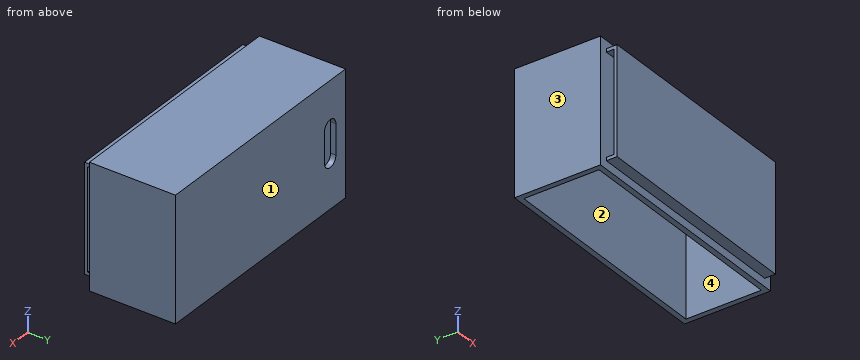
```python
from build123d import *

# Parameters (mm, degrees)
SKETCH3_W           = 55.88
SKETCH3_H           = 29.21
BOSS_EXTRUDE4_DEPTH = 20.32
SKETCH5_W           = 53.34
SKETCH5_H           = 17.78
CUT_EXTRUDE1_DEPTH  = 27.94
CUT_EXTRUDE2_REACH  = 22.32
SKETCH7_W           = 52.07
SKETCH7_H           = 25.4
BOSS_EXTRUDE5_DEPTH = 2.54
CUT_EXTRUDE3_REACH  = 55.975
SKETCH8_W           = 23.876
SKETCH8_H           = 1.778


with BuildPart() as part:
    # Sketch3 → Boss-Extrude4 (new body)
    with BuildSketch(Plane(origin=(0, 0, 0), x_dir=(1, 0, 0), z_dir=(0, 1, 0))):
        with Locations((27.94, 14.605)):
            Rectangle(SKETCH3_W, SKETCH3_H)
    extrude(amount=BOSS_EXTRUDE4_DEPTH)

    # Sketch5 → Cut-Extrude1 (cut)
    with BuildSketch(Plane(origin=(0, 0, -29.21), x_dir=(-1, 0, 0), z_dir=(0, 0, -1))):
        with Locations((-27.94, 10.16)):
            Rectangle(SKETCH5_W, SKETCH5_H)
    extrude(amount=-CUT_EXTRUDE1_DEPTH, mode=Mode.SUBTRACT)

    # Sketch6 → Cut-Extrude2 (cut, up to next)
    with BuildSketch(Plane(origin=(0, 20.32, 0), x_dir=(1, 0, 0), z_dir=(0, 1, 0)), mode=Mode.PRIVATE) as cut_extrude2_sk1:
        with BuildLine():
            Line((6.891061211, 17.925123576), (6.891061211, 10.769129072))
            ThreePointArc((6.891061211, 10.769129072), (5.021477061, 8.899544922), (3.151892912, 10.769129072))
            Line((3.151892912, 10.769129072), (3.151892912, 17.925123576))
            ThreePointArc((3.151892912, 17.925123576), (5.021477061, 19.794707726), (6.891061211, 17.925123576))
        make_face()
    cut_extrude2_tool1 = extrude(cut_extrude2_sk1.sketch, amount=-CUT_EXTRUDE2_REACH, mode=Mode.PRIVATE) & part.part
    add(cut_extrude2_tool1.solids().sort_by_distance((5.021477, 20.32, -14.347126))[0], mode=Mode.SUBTRACT)

    # Sketch7 → Boss-Extrude5 (add)
    with BuildSketch(Plane.XZ):
        with Locations((27.94, -14.605)):
            Rectangle(SKETCH7_W, SKETCH7_H)
    extrude(amount=BOSS_EXTRUDE5_DEPTH)

    # Sketch8 → Cut-Extrude3 (cut, up to next)
    with BuildSketch(Plane.ZY.offset(-1.905), mode=Mode.PRIVATE) as cut_extrude3_sk1:
        with Locations((-14.605, -0.889)):
            Rectangle(SKETCH8_W, SKETCH8_H)
    cut_extrude3_tool1 = extrude(cut_extrude3_sk1.sketch, amount=-CUT_EXTRUDE3_REACH, mode=Mode.PRIVATE) & part.part
    add(cut_extrude3_tool1.solids().sort_by_distance((1.905, -0.889, -14.605))[0], mode=Mode.SUBTRACT)


solid = part.part
```
The model under review builds one solid part; all positions refer to its coordinate system, in mm. Face numbers are marked on the shaded views. Round coordinates to 2 decimals unless told otherwise and drop trailing zeros. Order: outer loops, then holes, each group sorted by start corner. A loop starts at its lowest first (then second) coordinate and runs counter-clockwise, first axis right, second up. Notation, with made-up numbers: (34.5, 13.5) -> (84.5, 13.5) arc R20 ccw to (84.5, 23.5) -> close; hole circle Ø6 at (-34, 35.5). An arc over 180 degrees is marked (long way). Use a Markdown table: item, result.
Q1. Mouldability with a two-part tool opening along Y and no side actions: class the marked faces 1, 2, 3 and 4 as +Y half, -Y half, draft (parallel to the pull), parting line (faces both ways), or undercut.
Values:
| item | result |
|---|---|
| face 1 | +Y half |
| face 2 | undercut |
| face 3 | draft |
| face 4 | undercut |
Q2. We need section A-A on z = -5.25. Write out the cut boundary in (x, y) (3 decimals).
Values:
| item | result |
|---|---|
| outline | (0, 0) -> (55.88, 0) -> (55.88, 20.32) -> (0, 20.32) -> close; (1.905, -2.54) -> (53.975, -2.54) -> (53.975, -1.778) -> (1.905, -1.778) -> close; hole (1.27, 1.27) -> (54.61, 1.27) -> (54.61, 19.05) -> (1.27, 19.05) -> close |
Q3. For line 1 (Y direction, x = 38.5, z = -19.75); line 2 (X direction, y = 13.75, z = -18); line 3 (Y direction, x = 22.5, z = -1), list the stretches that pass through material, from the lowest coordinate up.
Values:
| item | result |
|---|---|
| line 1 | y = -2.54 to -1.78, 0 to 1.27, 19.05 to 20.32 |
| line 2 | x = 0 to 1.27, 54.61 to 55.88 |
| line 3 | y = 0 to 20.32 |
Q4. We need section C-C on z = -12.5. Write out the cut boundary in (x, y) (3 decimals), then the cut area to 3 significant figures.
Values:
| item | result |
|---|---|
| outline | (0, 0) -> (55.88, 0) -> (55.88, 20.32) -> (6.891, 20.32) -> (6.891, 19.05) -> (54.61, 19.05) -> (54.61, 1.27) -> (1.27, 1.27) -> (1.27, 19.05) -> (3.152, 19.05) -> (3.152, 20.32) -> (0, 20.32) -> close; (1.905, -2.54) -> (53.975, -2.54) -> (53.975, -1.778) -> (1.905, -1.778) -> close |
| area | 222 mm^2 |
Q5. We need section D-D on y = 4.5. Write out the cut boundary in (x, z).
Values:
| item | result |
|---|---|
| outline | (0, -29.21) -> (1.27, -29.21) -> (1.27, -1.27) -> (54.61, -1.27) -> (54.61, -29.21) -> (55.88, -29.21) -> (55.88, 0) -> (0, 0) -> close |
Q6. We need section B-B on x = 13. Write out the cut boundary in (y, z) (3 decimals), then the cut area to 3 significant figures.
Values:
| item | result |
|---|---|
| outline | (-2.54, -27.305) -> (0, -27.305) -> (0, -29.21) -> (1.27, -29.21) -> (1.27, -1.27) -> (19.05, -1.27) -> (19.05, -29.21) -> (20.32, -29.21) -> (20.32, 0) -> (0, 0) -> (0, -1.905) -> (-2.54, -1.905) -> close; hole (-1.778, -26.543) -> (0, -26.543) -> (0, -2.667) -> (-1.778, -2.667) -> close |
| area | 119 mm^2 |
Q7. Clearance check with flat-ended pins moving along their axes: P1, Ø3, axis at y = -2, z = -13, coming from the +X side (3 decimals); P2, Ø1.4, axis at x = 30.5, y = -1, coming from the -Z side (3 decimals); P3, Ø2, axis at y = -1.5, z = -17, coming from the -X side (3 decimals). State where each tip first meets the part, or that it passes through.
Values:
| item | result |
|---|---|
| P1 | stops at x = 53.975 |
| P2 | stops at z = -27.305 |
| P3 | stops at x = 1.905 |
